from build123d import *

# Parameters (mm, degrees)
SKETCH_1_W          = 19
SKETCH_1_H          = 19
SKETCH_1_W_2        = 13
SKETCH_1_H_2        = 13
EXTRUDE_1_DEPTH     = 95
SKETCH_2_R          = 1.65
CUT_EXTRUDE_1_DEPTH = 30
SKETCH_3_W          = 95
SKETCH_3_H          = 19
CUT_EXTRUDE_2_DEPTH = 16
SKETCH_4_W          = 53
SKETCH_4_H          = 12.7
EXTRUDE_1_2_DEPTH   = 2.9
CHAMFER_1_SIZE      = 2.5


with BuildPart() as part:
    # 草图1 → Extrude 1 (new body)
    with BuildSketch(Plane.XY):
        with Locations((6.5, 6.5)):
            Rectangle(SKETCH_1_W, SKETCH_1_H)
        with Locations((6.5, 6.5)):
            Rectangle(SKETCH_1_W_2, SKETCH_1_H_2, mode=Mode.SUBTRACT)
    extrude(amount=EXTRUDE_1_DEPTH)

    # 草图2 → 切除-拉伸1 (cut)
    with BuildSketch(Plane.ZY.offset(3)):
        with Locations((10, 6.5)):
            Circle(SKETCH_2_R)
        with Locations((85, 6.5)):
            Circle(SKETCH_2_R)
    extrude(amount=-CUT_EXTRUDE_1_DEPTH, mode=Mode.SUBTRACT)

    # 草图3 → 切除-拉伸2 (cut)
    with BuildSketch(Plane(origin=(16, 0, 0), x_dir=(0, 0, -1), z_dir=(1, 0, 0))):
        with Locations((-47.5, 6.5)):
            Rectangle(SKETCH_3_W, SKETCH_3_H)
    extrude(amount=-CUT_EXTRUDE_2_DEPTH, mode=Mode.SUBTRACT)

    # 草图4 → Extrude 1 2 (add)
    with BuildSketch(Plane(origin=(0, 0, 0), x_dir=(0, 0, -1), z_dir=(1, 0, 0))):
        with Locations((-47.5, 6.5)):
            Rectangle(SKETCH_4_W, SKETCH_4_H)
    extrude(amount=EXTRUDE_1_2_DEPTH)

    # 倒角1
    chamfer_1_edges = [part.edges().sort_by_distance(p)[0] for p in [
        (0, 6.5, 74),
        (0, 6.5, 21),
    ]]
    chamfer(chamfer_1_edges, length=CHAMFER_1_SIZE)


solid = part.part
Read the model definition and answer for the solid it produces. Units are mm, in the model's axes. A direction names the side the tool comes from. Give positions to 0.01 mm unless a question says otherwise; leave off trailing zeros. Loops run counter-clockwise (first coordinate to the right, second up) from the corner with the lowest first, then second, coordinate; pieces in that order, holes last. Notation, with made-up numbers: (32.25, -2.5) - (79.25, -2.5) arc R26 cw to (79.25, 34.5) - close; hole circle Ø6 at (8, -31). An arc over 180 degrees is marked (long way). Answer as CSV lines item,"result". Start each with the question number.
1) Find section B-B (z = 85). Write down the section's boundary in (x, y).
2) Determine the mould class of faces 3 (the face through (2.9, 7, 48)), 4 (the face through (-1.52, 6.57, 83.35)), 5 (the face through (1, 12.85, 48)), 6 (the face through (-2, -3, 47)) for opening direction Y: released by +Y, released by -Y, zero draft, split by the parting line, or undercut.
3) Find section C-C (z = 26.5). Write down the section's boundary in (x, y), then the cut area to 3 significant figures.
4) Find section A-A (y = 6.5). Write down the section's boundary in (x, z), then the cut area to 3 significant figures.
5) Find section D-D (y = 1.75). Write down the section's boundary in (x, z).
6) Straight lines are drawn through the part: L1, parallel to Y at x = -1, z = 10; L2, parallel to X at y = 3.75, z = 85; L3, parallel to Y at x = 1.2, z = 47.5. For each, find the intervals that lie inside material, in ascending order. Write a range as from..to.
7) Which of the six approach directions +Z, -Z, +X, -X, +Y, -Y give full straight-line access (tool end or side, diameter ignored) to faces 1 (the face through (1.3, 6.4, 75.2)), 2 (the face through (1, 0.15, 48))?
Findings below:
1,outline,"(-3, -3) - (0, -3) - (0, 4.85) - (-3, 4.85) - close; (-3, 8.15) - (0, 8.15) - (0, 16) - (-3, 16) - close"
2,face 3,"zero draft"
2,face 4,"undercut"
2,face 5,"released by +Y"
2,face 6,"released by -Y"
3,outline,"(-3, -3) - (0, -3) - (0, 0.15) - (2.9, 0.15) - (2.9, 12.85) - (0, 12.85) - (0, 16) - (-3, 16) - close"
3,area,"93.8 mm^2"
4,outline,"(-3, 0) - (0, 0) - (0, 8.35) - (-3, 8.35) - close; (-3, 11.65) - (0, 11.65) - (0, 18.5) - (2.5, 21) - (2.9, 21) - (2.9, 74) - (2.5, 74) - (0, 76.5) - (0, 83.35) - (-3, 83.35) - close; (-3, 86.65) - (0, 86.65) - (0, 95) - (-3, 95) - close"
4,area,"425 mm^2"
5,outline,"(-3, 0) - (0, 0) - (0, 18.5) - (2.5, 21) - (2.9, 21) - (2.9, 74) - (2.5, 74) - (0, 76.5) - (0, 95) - (-3, 95) - close"
6,L1,"-3..4.85, 8.15..16"
6,L2,"-3..0"
6,L3,"0.15..12.85"
7,face 1,"+Z, +X, +Y, -Y"
7,face 2,"+Z, -Z, +X, -Y"
